Source: three-view drawing plus pictorial views. Frame: mm from the lowest corner of the part. Give positions to 0.01 mm unless a question says otherwise; leave off trailing zeros. Write each loop counter-clockwise with the first axis right and the second up, starting at its lowest first coordinate (ties: lowest second). Pieces come first, ordered by that corner, then holes.
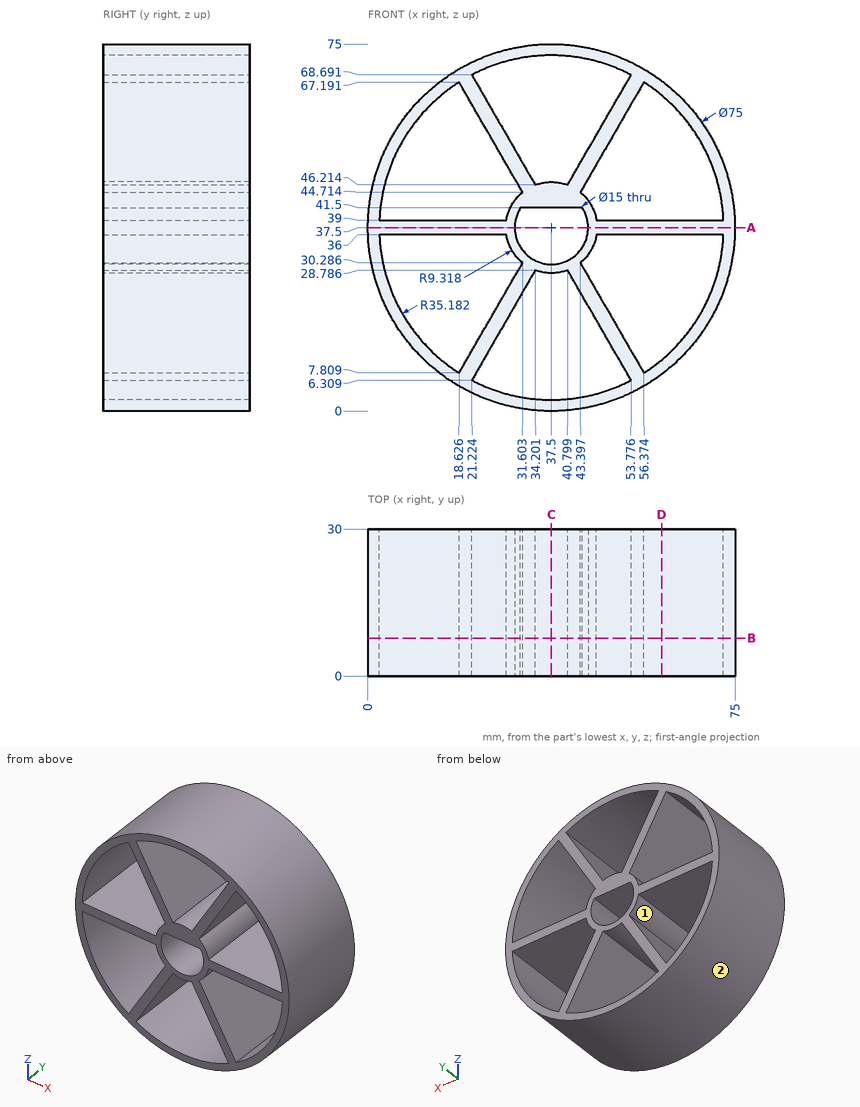
Q1. Pin query (flat end, axial travel): P1, Ø8, axis at x = 55.5, y = 11, coming from the -Z side; P2, Ø2, axis at y = 12, z = 62, coming from the +X side; P3, Ø8, axis at x = 66, y = 18, coming from the +Z side. Return the tip coordinate at first contact, or that it passes through.
Filled sheet:
P1: stops at z = 2.71
P2: stops at x = 66.72
P3: stops at z = 65.89
Q2. Section B-B on y = 7.75. Output: boundary loops of the cut face in (x, z), plus the area to 3 significant figures.
Filled sheet:
outline: circle Ø75 at (37.5, 37.5); hole (2.35, 36) arc R35.18 ccw to (18.63, 7.81) - (31.6, 30.29) arc R9.32 cw to (28.3, 36) - close; hole (2.35, 39) - (28.3, 39) arc R9.32 cw to (31.6, 44.71) - (18.63, 67.19) arc R35.18 ccw to start; hole (21.22, 6.31) arc R35.18 ccw to (53.78, 6.31) - (40.8, 28.79) arc R9.32 cw to (34.2, 28.79) - close; hole (21.22, 68.69) - (34.2, 46.21) arc R9.32 cw to (40.8, 46.21) - (53.78, 68.69) arc R35.18 ccw to start; hole (31.16, 41.5) arc R7.5 ccw (long way) to (43.84, 41.5) - close; hole (43.4, 30.29) - (56.37, 7.81) arc R35.18 ccw to (72.65, 36) - (46.7, 36) arc R9.32 cw to start; hole (43.4, 44.71) arc R9.32 cw to (46.7, 39) - (72.65, 39) arc R35.18 ccw to (56.37, 67.19) - close
area: 1,120 mm2
Q3. Ray query, line 1 along Z through (x, y) = (5.5, 22.75); line 2 along Z through (x, y) = (66, 22); line 3 along X through (y, z) = (10, 10) (1 decimal). Return the intervals inside material, ascending.
Filled sheet:
line 1: z = 17.95 to 22.88, 36 to 39, 52.12 to 57.05
line 2: z = 13.13 to 16.87, 36 to 39, 58.13 to 61.87
line 3: x = 12 to 15.6, 19.9 to 23.4, 51.6 to 55.1, 59.4 to 63
Q4. Section C-C on x = 37.5. Output: boundary loops of the cut face in (y, z), plus the area to 3 significant figures.
Filled sheet:
outline: (0, 0) - (30, 0) - (30, 2.32) - (0, 2.32) - close; (0, 28.18) - (30, 28.18) - (30, 30) - (0, 30) - close; (0, 41.5) - (30, 41.5) - (30, 46.82) - (0, 46.82) - close; (0, 72.68) - (30, 72.68) - (30, 75) - (0, 75) - close
area: 353 mm2
Q5. Section D-D on x = 60. Output: boundary loops of the cut face in (y, z).
Filled sheet:
outline: (0, 7.5) - (30, 7.5) - (30, 10.45) - (0, 10.45) - close; (0, 36) - (30, 36) - (30, 39) - (0, 39) - close; (0, 64.55) - (30, 64.55) - (30, 67.5) - (0, 67.5) - close
Q6. Pull-direction query (X, two-part tool) for the marked faces 1 and 2; classes: released by +X, released by -X, zero draft, split by the parting line, or undercut.
Filled sheet:
face 1: undercut
face 2: split by the parting line
Q7. Section A-A on z = 37.5. Output: boundary loops of the cut face in (x, y).
Filled sheet:
outline: (0, 0) - (30, 0) - (30, 30) - (0, 30) - close; (45, 0) - (75, 0) - (75, 30) - (45, 30) - close
